Geometry check sheet. Reference: the model listing, model coordinates, mm. A direction names the side the tool comes from. Round coordinates to 2 decimals unless told otherwise and drop trailing zeros. Order: outer loops, then holes, each group sorted by start corner. A loop starts at its lowest first (then second) coordinate and runs counter-clockwise, first axis right, second up. Notation, with made-up numbers: (-28.5, 54) - (-9.5, 54) arc R13 ccw to (-9.5, 76) - close; hole circle Ø11 at (23.5, 65). An arc over 180 degrees is marked (long way). Write each question's results on one line, items separated by ' | '.
```python
from build123d import *

# Parameters (mm, degrees)
F1_DEPTH = 76.2
F3_DEPTH = 104.776
F4_DEPTH = 104.776
F5_W     = 6.35
F5_H     = 19.05
F6_DEPTH = 73.026
F7_W     = 6.35
F7_H     = 19.05
F8_DEPTH = 73.026


with BuildPart() as f1:
    # F0 (on Front) → F1 (new body)
    with BuildSketch(Plane.XZ):
        Polygon((0, -50.8), (0, 0), (19.05, 50.8), (69.85, 50.8), (69.85, 53.975), (16.849724, 53.975), (-3.175, 0.575737), (-3.175, -50.8), align=None)
    extrude(amount=F1_DEPTH)

    # F2 (on face) → F3 (cut, through all)
    with BuildSketch(Plane.XY.offset(53.975)):
        with BuildLine():
            ThreePointArc((53.975, -19.05), (56.220064, -18.120064), (57.15, -15.875))
            ThreePointArc((57.15, -15.875), (56.220064, -13.629936), (53.975, -12.7))
            ThreePointArc((53.975, -12.7), (50.8, -15.875), (53.975, -19.05))
        make_face()
        with BuildLine():
            ThreePointArc((53.975, -19.05), (50.8, -15.875), (53.975, -12.7))
            Line((53.975, -12.7), (34.925, -12.7))
            ThreePointArc((34.925, -12.7), (37.170064, -13.629936), (38.1, -15.875))
            ThreePointArc((38.1, -15.875), (37.170064, -18.120064), (34.925, -19.05))
            Line((34.925, -19.05), (53.975, -19.05))
        make_face()
        with BuildLine():
            ThreePointArc((38.1, -15.875), (37.170064, -13.629936), (34.925, -12.7))
            ThreePointArc((34.925, -12.7), (31.75, -15.875), (34.925, -19.05))
            ThreePointArc((34.925, -19.05), (37.170064, -18.120064), (38.1, -15.875))
        make_face()
    extrude(amount=-F3_DEPTH, mode=Mode.SUBTRACT)

    # F2 (on face) → F4 (cut, through all)
    with BuildSketch(Plane.XY.offset(53.975)):
        with BuildLine():
            ThreePointArc((38.1, -60.325), (37.170064, -58.079936), (34.925, -57.15))
            ThreePointArc((34.925, -57.15), (31.75, -60.325), (34.925, -63.5))
            ThreePointArc((34.925, -63.5), (37.170064, -62.570064), (38.1, -60.325))
        make_face()
        with BuildLine():
            ThreePointArc((53.975, -63.5), (56.220064, -62.570064), (57.15, -60.325))
            ThreePointArc((57.15, -60.325), (56.220064, -58.079936), (53.975, -57.15))
            ThreePointArc((53.975, -57.15), (50.8, -60.325), (53.975, -63.5))
        make_face()
        with BuildLine():
            ThreePointArc((53.975, -63.5), (50.8, -60.325), (53.975, -57.15))
            Line((53.975, -57.15), (34.925, -57.15))
            ThreePointArc((34.925, -57.15), (37.170064, -58.079936), (38.1, -60.325))
            ThreePointArc((38.1, -60.325), (37.170064, -62.570064), (34.925, -63.5))
            Line((34.925, -63.5), (53.975, -63.5))
        make_face()
    extrude(amount=-F4_DEPTH, mode=Mode.SUBTRACT)

    # F5 (on face) → F6 (cut, through all)
    with BuildSketch(Plane(origin=(-3.175, 0, 0), x_dir=(0, -1, 0), z_dir=(-1, 0, 0))):
        with BuildLine():
            Line((19.05, -34.925), (12.7, -34.925))
            ThreePointArc((12.7, -34.925), (15.875, -38.1), (19.05, -34.925))
        make_face()
        with BuildLine():
            ThreePointArc((19.05, -15.875), (15.875, -12.7), (12.7, -15.875))
            Line((12.7, -15.875), (19.05, -15.875))
        make_face()
        with Locations((15.875, -25.4)):
            Rectangle(F5_W, F5_H)
    extrude(amount=-F6_DEPTH, mode=Mode.SUBTRACT)

    # F7 (on face) → F8 (cut, through all)
    with BuildSketch(Plane(origin=(-3.175, 0, 0), x_dir=(0, -1, 0), z_dir=(-1, 0, 0))):
        with BuildLine():
            Line((57.15, -15.875), (63.5, -15.875))
            ThreePointArc((63.5, -15.875), (60.325, -12.7), (57.15, -15.875))
        make_face()
        with BuildLine():
            ThreePointArc((57.15, -34.925), (60.325, -38.1), (63.5, -34.925))
            Line((63.5, -34.925), (57.15, -34.925))
        make_face()
        with Locations((60.325, -25.4)):
            Rectangle(F7_W, F7_H)
    extrude(amount=-F8_DEPTH, mode=Mode.SUBTRACT)


solid = f1.part
```
(1) Section check C-C (y = -59). Record the cut outline in (x, z) (3 decimals), then the cut area to 3 significant figures.
Answers follow:
outline: (-3.175, -50.8) - (0, -50.8) - (0, -37.81) - (-3.175, -37.81) - close; (-3.175, -12.99) - (0, -12.99) - (0, 0) - (19.05, 50.8) - (32.04, 50.8) - (32.04, 53.975) - (16.85, 53.975) - (-3.175, 0.576) - close; (56.86, 50.8) - (69.85, 50.8) - (69.85, 53.975) - (56.86, 53.975) - close | area: 346 mm²
(2) Depth check by flat-ended pin: pin 1 Ø8 at (x, y) = (44, -25.5) entering from -Z; pin 2 Ø15 at (y, z) = (-35, -20) entering from +X; pin 3 Ø4 at (y, z) = (-54.5, 35.5) entering from +X. Enter the tip coordinate at first touch or a pass-through.
Answers follow:
pin 1: z = 50.8 | pin 2: x = 0 | pin 3: x = 14.06
(3) Material ranges on line 1 (Z direction, x = 24.5, y = -7.5) (3 decimals); line 2 (X direction, y = -57.5, z = -37.5) (3 decimals); line 3 (X direction, y = -64.5, z = 6.5), recorded low to high.
Answers follow:
line 1: 50.8 to 53.975 | line 2: -3.175 to 0 | line 3: -0.95 to 2.44
(4) Section check A-A (z = -25). Record the cut outline in (x, y) (3 decimals).
Answers follow:
outline: (-3.175, -76.2) - (0, -76.2) - (0, -63.5) - (-3.175, -63.5) - close; (-3.175, -57.15) - (0, -57.15) - (0, -19.05) - (-3.175, -19.05) - close; (-3.175, -12.7) - (0, -12.7) - (0, 0) - (-3.175, 0) - close
(5) Section check B-B (x = 50). Record the cut outline in (y, z) (3 decimals).
Answers follow:
outline: (-76.2, 50.8) - (-63.5, 50.8) - (-63.5, 53.975) - (-76.2, 53.975) - close; (-57.15, 50.8) - (-19.05, 50.8) - (-19.05, 53.975) - (-57.15, 53.975) - close; (-12.7, 50.8) - (0, 50.8) - (0, 53.975) - (-12.7, 53.975) - close
(6) Section check D-D (y = -70.5). Record the cut outline in (x, z) (3 decimals).
Answers follow:
outline: (-3.175, -50.8) - (0, -50.8) - (0, 0) - (19.05, 50.8) - (69.85, 50.8) - (69.85, 53.975) - (16.85, 53.975) - (-3.175, 0.576) - close
(7) Access from +Z, -Z, +X, -X, +Y, -Y to the whole of each face (thin tool, end or side, straight path). Record for faces 5 (the face through (31.75, -15.81, 52.41)), 6 (the face through (69.85, -38, 52)), 7 (the face through (-2, -57.15, -26)), 8 (the face through (44, -38, 50.8)).
Answers follow:
face 5: +Z, -Z | face 6: +Z, -Z, +X, +Y, -Y | face 7: +X, -X | face 8: -Z, +X, +Y, -Y
(8) Draft check along Z on faces 1 (the face through (-2, -63.5, -26)), 2 (the face through (-2, -12.7, -26)), 3 (the face through (9.39, -37.57, 25.04)), 4 (the face through (31.75, -60.26, 52.41)). Enter one of: released by +Z, released by -Z, zero draft, split by the parting line, or undercut.
Answers follow:
face 1: undercut | face 2: undercut | face 3: released by -Z | face 4: zero draft
